Build history of the part. All positions in model axes, mm. A direction names the side the tool comes from. Round coordinates to 2 decimals unless told otherwise and drop trailing zeros. One line per question, with ' | ' between items. Start each with the question number.
from build123d import *

# Parameters (mm, degrees)
SKETCH1_R                  = 93.345
BASE_DEPTH                 = 4.7625
BASE_DEPTH_BACK            = 4.7625
BOTTOM_SUPPORT_HOLES_DEPTH = 10.525
BOTTOM_SUPPORT_GUIDE_DEPTH = 12.7
SKETCH6_R                  = 1.27
BOTTOM_BOLT_HOLE_DEPTH     = 12.7
TOP_SUPPORT_HOLES_DEPTH    = 4.7625
TOP_SUPPORT_GUIDE_DEPTH    = 12.7
SKETCH12_R                 = 1.27
TOP_BOLT_HOLE_DEPTH        = 12.7
BOTTOM_PATTERN_COUNT       = 4
CIRPATTERN3_COUNT          = 4
SKETCH13_R                 = 34.925
CUT_EXTRUDE5_DEPTH         = 12.7


with BuildPart() as part:
    # Sketch1 → Base (new body, two sides)
    with BuildSketch(Plane(origin=(0, 0, 0), x_dir=(1, 0, 0), z_dir=(0, 1, 0))) as base_sk:
        Circle(SKETCH1_R)
    extrude(amount=BASE_DEPTH)
    extrude(base_sk.sketch, amount=-BASE_DEPTH_BACK)

    # Sketch2 → Bottom support holes (cut, through all)
    with BuildSketch(Plane(origin=(0, 4.7625, 0), x_dir=(1, 0, 0), z_dir=(0, 1, 0))):
        with BuildLine():
            Line((0, 88.9), (0, 83.82))
            ThreePointArc((0, 83.82), (-21.72026739, 80.956916842), (-41.956713931, 72.563258996))
            Line((-41.956713931, 72.563258996), (-44.39288973, 77.022602796))
            ThreePointArc((-44.39288973, 77.022602796), (-22.977169228, 85.879332172), (0, 88.9))
        make_face()
    bottom_support_holes = extrude(amount=-BOTTOM_SUPPORT_HOLES_DEPTH, mode=Mode.SUBTRACT)

    # Sketch3 → Bottom support guide (add)
    with BuildSketch(Plane(origin=(0, 4.7625, 0), x_dir=(1, 0, 0), z_dir=(0, 1, 0))):
        with BuildLine():
            Line((0, 83.82), (0, 76.2))
            ThreePointArc((0, 76.2), (-19.834896001, 73.573207764), (-38.302281481, 65.8739344))
            Line((-38.302281481, 65.8739344), (-41.956713931, 72.563258996))
            ThreePointArc((-41.956713931, 72.563258996), (-21.72026739, 80.956916842), (0, 83.82))
        make_face()
    bottom_support_guide = extrude(amount=BOTTOM_SUPPORT_GUIDE_DEPTH)

    # Sketch6 → Bottom bolt hole (cut, symmetric)
    with BuildSketch(Plane(origin=(-20.978356966, 0, -78.191629498), x_dir=(-0.965842482, 0, 0.25912989), z_dir=(-0.25912989, 0, -0.965842482))):
        with Locations((-0.00326739, 11.1125)):
            Circle(SKETCH6_R)
    bottom_bolt_hole = extrude(amount=BOTTOM_BOLT_HOLE_DEPTH, both=True, mode=Mode.SUBTRACT)

    # Sketch8 → Top support holes (cut)
    with BuildSketch(Plane(origin=(-31.122978549, 4.7625, 77.296707326), x_dir=(1, 0, 0), z_dir=(0, 1, 0))):
        with BuildLine():
            Line((-31.738814298, 140.158500173), (-28.14671185, 136.566397725))
            ThreePointArc((-28.14671185, 136.566397725), (-41.480754694, 119.183343848), (-49.854870889, 98.93880289))
            Line((-49.854870889, 98.93880289), (-54.730739557, 100.369398703))
            ThreePointArc((-54.730739557, 100.369398703), (-45.850191767, 121.775253295), (-31.738814298, 140.158500173))
        make_face()
    top_support_holes = extrude(amount=-TOP_SUPPORT_HOLES_DEPTH, mode=Mode.SUBTRACT)

    # Sketch10 → Top support guide (add)
    with BuildSketch(Plane(origin=(-31.122978549, 4.7625, 77.296707326), x_dir=(1, 0, 0), z_dir=(0, 1, 0))):
        with BuildLine():
            Line((-28.14671185, 136.566397725), (-22.758558177, 131.178244052))
            ThreePointArc((-22.758558177, 131.178244052), (-34.92652504, 115.295431983), (-42.540730139, 96.792810073))
            Line((-42.540730139, 96.792810073), (-49.854870889, 98.93880289))
            ThreePointArc((-49.854870889, 98.93880289), (-41.480754694, 119.183343848), (-28.14671185, 136.566397725))
        make_face()
    top_support_guide = extrude(amount=TOP_SUPPORT_GUIDE_DEPTH)

    # Sketch12 → Top bolt hole (cut, symmetric)
    with BuildSketch(Plane(origin=(-70.123769919, 0, -40.455892982), x_dir=(-0.499721266, 0, 0.866186271), z_dir=(-0.866186271, 0, -0.499721266))):
        with Locations((-0.00326739, 11.1125)):
            Circle(SKETCH12_R)
    top_bolt_hole = extrude(amount=TOP_BOLT_HOLE_DEPTH, both=True, mode=Mode.SUBTRACT)

    # Bottom pattern: Bottom support holes, Bottom support guide, Bottom bolt hole ×4 about axis
    bottom_pattern_axis = Axis((0, 0, 0), (0, 1, 0))
    for i in range(1, BOTTOM_PATTERN_COUNT):
        add(bottom_support_holes.rotate(bottom_pattern_axis, i * 360 / BOTTOM_PATTERN_COUNT), mode=Mode.SUBTRACT)
        add(bottom_support_guide.rotate(bottom_pattern_axis, i * 360 / BOTTOM_PATTERN_COUNT))
        add(bottom_bolt_hole.rotate(bottom_pattern_axis, i * 360 / BOTTOM_PATTERN_COUNT), mode=Mode.SUBTRACT)

    # CirPattern3: Top support holes, Top support guide, Top bolt hole ×4 about axis
    cirpattern3_axis = Axis((0, 0, 0), (0, 1, 0))
    for i in range(1, CIRPATTERN3_COUNT):
        add(top_support_holes.rotate(cirpattern3_axis, i * 360 / CIRPATTERN3_COUNT), mode=Mode.SUBTRACT)
        add(top_support_guide.rotate(cirpattern3_axis, i * 360 / CIRPATTERN3_COUNT))
        add(top_bolt_hole.rotate(cirpattern3_axis, i * 360 / CIRPATTERN3_COUNT), mode=Mode.SUBTRACT)

    # Sketch13 → Cut-Extrude5 (cut)
    with BuildSketch(Plane(origin=(0, 4.7625, 0), x_dir=(1, 0, 0), z_dir=(0, 1, 0))):
        Circle(SKETCH13_R)
    extrude(amount=-CUT_EXTRUDE5_DEPTH, mode=Mode.SUBTRACT)

    # Sketch14 → Cut-Revolve1 (revolve, cut)
    with BuildSketch(Plane.XY):
        Polygon((34.925, 4.7625), (34.925, -4.7625), (53.618865065, 4.7625), align=None)
    revolve(axis=Axis((0, 25.4, 0), (0, -1, 0)), mode=Mode.SUBTRACT)


solid = part.part
Item 1: Two-plate mould, pull along Z, no slides. Class faces 1 (the face through (50.18, 0.07, -78.71)), 2 (the face through (43.158, 0.067, 74.762)), 3 (the face through (-20.554, 11.024, 77.27)): +Z half, -Z half, draft (parallel to the pull), parting line (faces both ways), or undercut.
Item 2: Flat gauge pins, fed straight in: pin 1 (8.5 mm diameter, centred on x = -79.5, y = 12, fed in from -Z); pin 2 (13.5 mm diameter, centred on x = 79, z = 41, fed in from +Y); pin 3 (5.5 mm diameter, centred on x = -87, y = -1, fed in from +Z); pin 4 (12 mm diameter, centred on x = 70.5, y = 11, fed in from +Z). Where does each tip first touch, or does it go through?
Item 3: Tool access for faces 4 (the face through (74.762, 0.067, -43.158)), 5 (the face through (69.172, 11.024, -40.104)), 6 (the face through (83.382, 2.415, 22.347)): list every direction of +Z, -Z, +X, -X, +Y, -Y with a clear straight run to the whole face (end or side of a thin tool).
Item 4: Cut at A-A on y = 15. Count the separate pieces of the cut face and the enclosed holes in it, then the cut area to 3 significant figures.
Item 5: Wall check: line 1 along X through (y, z) = (-0.5, 10); line 2 along Z through (x, y) = (21.5, -0.5); line 3 along Y through (x, z) = (72, 54). Give the ranges that are in metal, low to high. Write a range as [from, to].
Results found:
1) face 1: parting line | face 2: undercut | face 3: +Z half
2) pin 1: stops at z = -36.92 | pin 2: stops at y = 17.46 | pin 3: stops at z = 40.19 | pin 4: stops at z = 53.53
3) face 4: +Y, -Y | face 5: -Z, +Y | face 6: +Y
4) separate pieces: 8 | enclosed holes: 0 | area: 2,560 mm^2
5) line 1: x = [-92.81, -88.34], [-83.22, -42.12], [42.12, 92.81] | line 2: z = [-90.84, -37.57], [37.57, 81.02], [86.26, 90.84] | line 3: y = [-4.76, 4.76]
